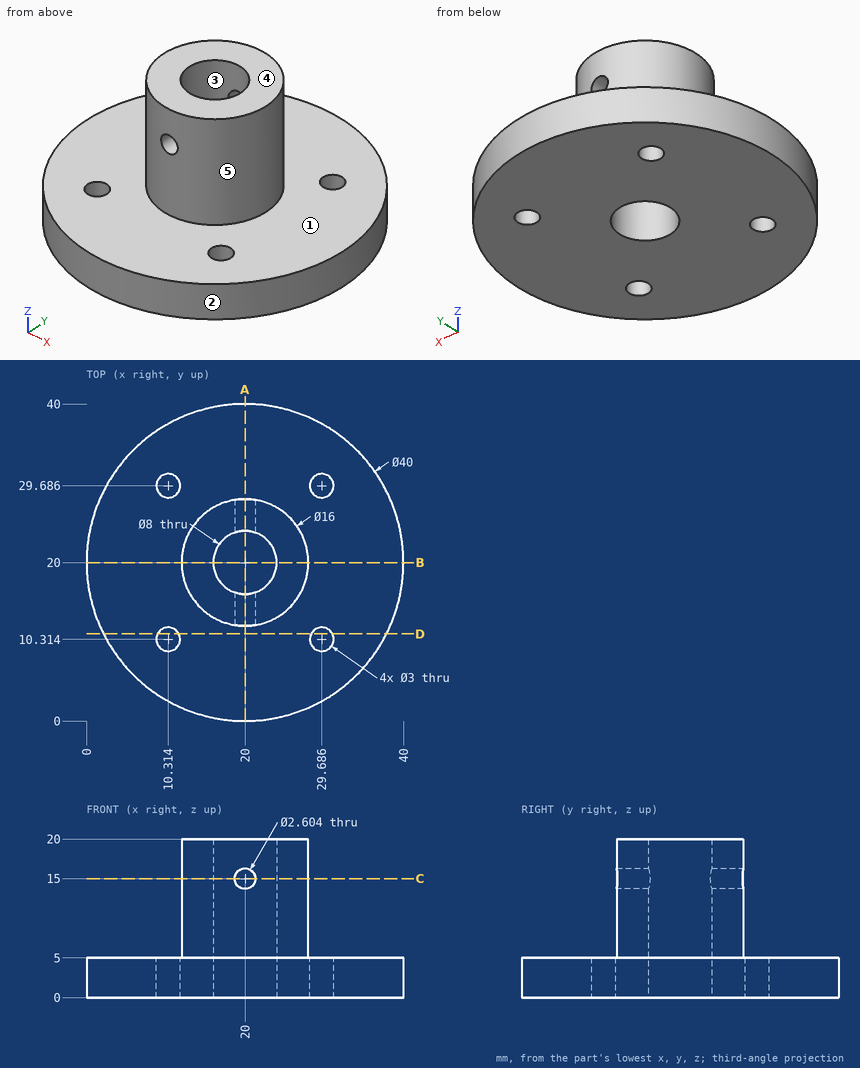
Check sheet for the drawn part. Datum: minimum x, y, z corner. Units: mm. A direction names the side the tool comes from. Round coordinates to 2 decimals unless told otherwise and drop trailing zeros. Write each loop counter-clockwise with the first axis right and the second up, starting at its lowest first coordinate (ties: lowest second). Pieces come first, ordered by that corner, then holes. Notation, with made-up numbers: (44, -25.5) - (71, -25.5) arc R19 ccw to (71, 5.5) - close; hole circle Ø10 at (32.25, 17). An arc over 180 degrees is marked (long way). Write each question's results on one line, items separated by ' | '.
(1) Depth check by flat-ended pin: pin 1 Ø1 at (x, z) = (20, 7.5) entering from -Y; pin 2 Ø1.8 at (x, y) = (29.69, 29.69) entering from -Z; pin 3 Ø5 at (y, z) = (28.5, 13) entering from +X; pin 4 Ø1 at (x, z) = (26.5, 16) entering from +Y. Enter the tip coordinate at first touch or a pass-through.
Computed:
pin 1: stops at y = 12 | pin 2: passes through | pin 3: stops at x = 25.29 | pin 4: stops at y = 25.29
(2) Set-up check for the marked faces 1 and 2: record each of +Z, -Z, +X, -X, +Y, -Y from which the full face is reachable in a straight line by a thin tool's end or side.
Computed:
face 1: +Z | face 2: +Z, -Z
(3) Draft check along Y on the marked faces 3, 4 and 5. Enter one of: pulls with the +Y half, pulls with the -Y half, needs draft (parallel to the pull), parting line crosses it, or undercut.
Computed:
face 3: undercut | face 4: needs draft | face 5: parting line crosses it
(4) Sectioned sample at C-C, the plane z = 15. Enter the section's corners in (x, y), plus the area to 3 significant figures.
Computed:
outline: (18.7, 12.11) - (18.7, 16.22) arc R4 cw to (18.7, 23.78) - (18.7, 27.89) arc R8 ccw to start; (21.3, 12.11) arc R8 ccw to (21.3, 27.89) - (21.3, 23.78) arc R4 cw to (21.3, 16.22) - close | area: 130 mm^2
(5) Sectioned sample at D-D, the plane y = 11. Enter the section's corners in (x, z).
Computed:
outline: (2.14, 0) - (8.98, 0) - (8.98, 5) - (2.14, 5) - close; (11.65, 0) - (28.35, 0) - (28.35, 5) - (11.65, 5) - close; (31.02, 0) - (37.86, 0) - (37.86, 5) - (31.02, 5) - close
(6) Sectioned sample at B-B, the plane y = 20. Enter the section's corners in (x, z).
Computed:
outline: (0, 0) - (16, 0) - (16, 20) - (12, 20) - (12, 5) - (0, 5) - close; (24, 0) - (40, 0) - (40, 5) - (28, 5) - (28, 20) - (24, 20) - close
(7) Thickness scan on probe 1 along Y at (x, z) = (20, 12.5); probe 2 along Z at (x, y) = (25, 30.5); probe 3 along Y at (x, z) = (23.5, 16.5) (1 decimal). Record the ranges inside material, lowest first. Write a range as from..to.
Computed:
probe 1: y = 12..16, 24..28 | probe 2: z = 0..5 | probe 3: y = 12.8..18.1, 21.9..27.2
(8) Sectioned sample at A-A, the plane x = 20. Enter the section's corners in (y, z), plus the area to 3 significant figures.
Computed:
outline: (0, 0) - (16, 0) - (16, 13.7) - (12, 13.7) - (12, 5) - (0, 5) - close; (12, 16.3) - (16, 16.3) - (16, 20) - (12, 20) - close; (24, 0) - (40, 0) - (40, 5) - (28, 5) - (28, 13.7) - (24, 13.7) - close; (24, 16.3) - (28, 16.3) - (28, 20) - (24, 20) - close | area: 259 mm^2
